Can you work these out from the drawing? Everything is in mm from the part's minimum corner. A direction names the side the tool comes from. Coordinates: 2 decimals unless noted, no trailing zeros. Order: outer loops, then holes, each group sorted by start corner. A loop starts at its lowest first (then second) coordinate and runs counter-clockwise, first axis right, second up. Notation, with made-up numbers: M 66,43.5 L 83,43.5 A6 ccw 83,48.5 Z; hole C 81.25,63 d11. An arc over 180 degrees is marked long. Answer as a JSON object with one key per item and string values.
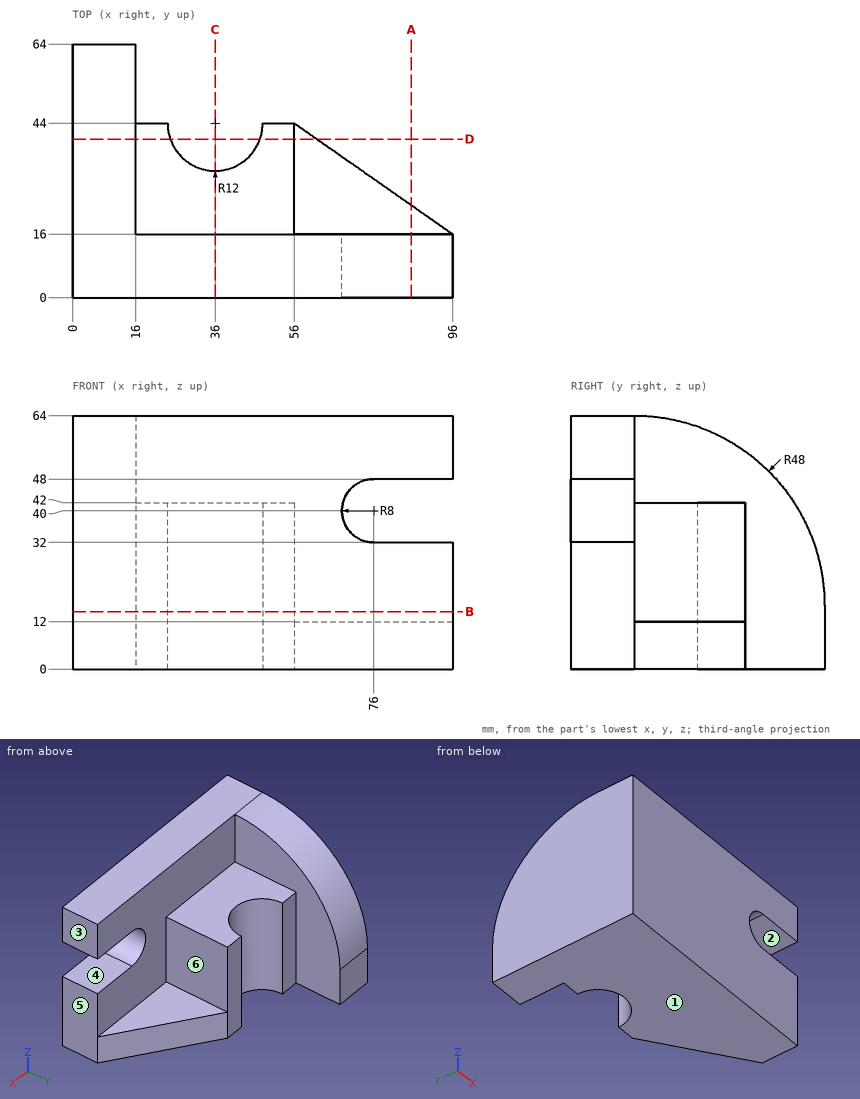
Item 1: Please list where these lines run through material, in increasing order: line 1 (X direction, y = 27.5, z = 36); line 2 (Z direction, x = 63.5, y = 19); line 3 (X direction, y = 36, z = 29).
Answers follow:
{"line 1": "x = 0 to 56", "line 2": "z = 0 to 12", "line 3": "x = 0 to 27.06, 44.94 to 56"}
Item 2: I want a section at D-D, the plane y = 40. Write out the boundary of the cut face in (x, z), plus the area to 3 significant figures.
Answers follow:
{"outline": "M 0,0 L 24.69,0 L 24.69,42 L 16,42 L 16,57.57 L 0,57.57 Z; M 47.31,0 L 61.71,0 L 61.71,12 L 56,12 L 56,42 L 47.31,42 Z", "area": "1,720 mm^2"}
Item 3: If we mould it in two halves opening along Z, with no side actions, what happens to the marked faces 1, 2, 3 and 4? For each: pulls with the +Z half, pulls with the -Z half, needs draft (parallel to the pull), parting line crosses it, or undercut.
Answers follow:
{"face 1": "pulls with the -Z half", "face 2": "undercut", "face 3": "needs draft", "face 4": "undercut"}
Item 4: I'm going to push flat-ended pins straight in: pin 1 (2.5 mm diameter, centred on x = 19.5, z = 19.5, fed in from +Y); pin 2 (5 mm diameter, centred on y = 53.5, z = 42.5, fed in from +X); pin 3 (3 mm diameter, centred on x = 64.5, y = 31.5, fed in from +Z). Where does each tip first touch, or does it pass through?
Answers follow:
{"pin 1": "stops at y = 44", "pin 2": "stops at x = 16", "pin 3": "stops at z = 12"}
Item 5: I want a section at C-C, the plane x = 36. Write out the boundary of the cut face in (y, z).
Answers follow:
{"outline": "M 0,0 L 32,0 L 32,42 L 16,42 L 16,64 L 0,64 Z"}
Item 6: Which directions (+Z, -Z, +X, -X, +Y, -Y) give clear straight access to the entire face, cutting with the end or side of a thin tool? Please do the marked faces 5 and 6.
Answers follow:
{"face 5": "+Z, -Z, +X, +Y, -Y", "face 6": "+Z, +X, +Y"}
Item 7: I want a section at A-A, the plane x = 85.5. Write out the boundary of the cut face in (y, z).
Answers follow:
{"outline": "M 0,0 L 23.35,0 L 23.35,12 L 16,12 L 16,32 L 0,32 Z; M 0,48 L 16,48 L 16,64 L 0,64 Z"}
Item 8: I want a section at B-B, the plane z = 14.5. Write out the boundary of the cut face in (x, y), plus the area to 3 significant figures.
Answers follow:
{"outline": "M 0,0 L 96,0 L 96,16 L 56,16 L 56,44 L 48,44 A12 cw 24,44 L 16,44 L 16,64 L 0,64 Z", "area": "3,200 mm^2"}
